Design review of the part built by this model. Coordinates are the model's own, in mm. Give positions to 0.01 mm unless a question says otherwise; leave off trailing zeros. Loops run counter-clockwise (first coordinate to the right, second up) from the corner with the lowest first, then second, coordinate; pieces in that order, holes last. Notation, with made-up numbers: (-5.75, 73.5) -> (42.25, 73.5) arc R22 cw to (42.25, 98.5) -> close; hole circle Ø5 at (-12, -4). An arc over 180 degrees is marked (long way). Use a Markdown table: item, result. Add a question column.
1. To check wall thickness, follow line 1 (X direction, y = 109, z = 10.1); line 2 (Z direction, x = 10.5, y = 164.5); line 3 (X direction, y = 16, z = 9). State the ranges of each line that lie inside material, in increasing order.
2. Add section D-D (y = 158). Count the separate pieces of the cut face and the enclosed holes in it, and give its area (3 significant figures).
3. Add section C-C (x = -10.1). State the section outline as (y, z) points.
4. Add section B-B (z = 10.1). State the section outline as (x, y) points, and give its area (3 significant figures).
5. Add section A-A (x = 0). State the section outline as (y, z) points, and give its area (3 significant figures).
6. For pin 1 Ø8 at (x, z) = (10.1, -10.1) entering from +Y; pin 2 Ø0.7 at (x, y) = (-14.5, 79.5) entering from +Z, all flat-tipped, find the tip position at first contact; note any pin that passes through.
```python
from build123d import *

# Parameters (mm, degrees)
SKETCH_1_R      = 2.5
SKETCH_1_R_2    = 3.4
EXTRUDE_1_DEPTH = 181


with BuildPart() as part:
    # 草图1 → 凸台-拉伸1 (new body)
    with BuildSketch(Plane(origin=(0, 0, 0), x_dir=(1, 0, 0), z_dir=(0, 1, 0))):
        with BuildLine():
            Line((-14, 15), (-3.25, 15))
            Line((-3.25, 15), (-3.25, 12.7))
            Line((-3.25, 12.7), (-5.2, 12.7))
            Line((-5.2, 12.7), (-5.2, 6.9))
            ThreePointArc((-5.2, 6.9), (0, 4.3), (5.2, 6.9))
            Line((5.2, 6.9), (5.2, 12.7))
            Line((5.2, 12.7), (3.25, 12.7))
            Line((3.25, 12.7), (3.25, 15))
            Line((3.25, 15), (14, 15))
            ThreePointArc((14, 15), (14.707106781, 14.707106781), (15, 14))
            Line((15, 14), (15, 3.25))
            Line((15, 3.25), (12.7, 3.25))
            Line((12.7, 3.25), (12.7, 5.2))
            Line((12.7, 5.2), (6.9, 5.2))
            ThreePointArc((6.9, 5.2), (4.3, 0), (6.9, -5.2))
            Line((6.9, -5.2), (12.7, -5.2))
            Line((12.7, -5.2), (12.7, -3.25))
            Line((12.7, -3.25), (15, -3.25))
            Line((15, -3.25), (15, -14))
            ThreePointArc((15, -14), (14.707106781, -14.707106781), (14, -15))
            Line((14, -15), (3.25, -15))
            Line((3.25, -15), (3.25, -12.7))
            Line((3.25, -12.7), (5.2, -12.7))
            Line((5.2, -12.7), (5.2, -6.9))
            ThreePointArc((5.2, -6.9), (0, -4.3), (-5.2, -6.9))
            Line((-5.2, -6.9), (-5.2, -12.7))
            Line((-5.2, -12.7), (-3.25, -12.7))
            Line((-3.25, -12.7), (-3.25, -15))
            Line((-3.25, -15), (-14, -15))
            ThreePointArc((-14, -15), (-14.707106781, -14.707106781), (-15, -14))
            Line((-15, -14), (-15, -3.25))
            Line((-15, -3.25), (-12.7, -3.25))
            Line((-12.7, -3.25), (-12.7, -5.2))
            Line((-12.7, -5.2), (-6.9, -5.2))
            ThreePointArc((-6.9, -5.2), (-4.3, 0), (-6.9, 5.2))
            Line((-6.9, 5.2), (-12.7, 5.2))
            Line((-12.7, 5.2), (-12.7, 3.25))
            Line((-12.7, 3.25), (-15, 3.25))
            Line((-15, 3.25), (-15, 14))
            ThreePointArc((-15, 14), (-14.707106781, 14.707106781), (-14, 15))
        make_face()
        with Locations(Location((0, 0, 0), (0, 0, 270))):
            Circle(SKETCH_1_R, mode=Mode.SUBTRACT)
        with Locations(Location((-10.1, 10.1, 0), (0, 0, 270))):
            Circle(SKETCH_1_R_2, mode=Mode.SUBTRACT)
        with Locations(Location((10.1, 10.1, 0), (0, 0, 90))):
            Circle(SKETCH_1_R_2, mode=Mode.SUBTRACT)
        with Locations(Location((10.1, -10.1, 0), (0, 0, 270))):
            Circle(SKETCH_1_R_2, mode=Mode.SUBTRACT)
        with Locations(Location((-10.1, -10.1, 0), (0, 0, 90))):
            Circle(SKETCH_1_R_2, mode=Mode.SUBTRACT)
    extrude(amount=EXTRUDE_1_DEPTH)


solid = part.part
```
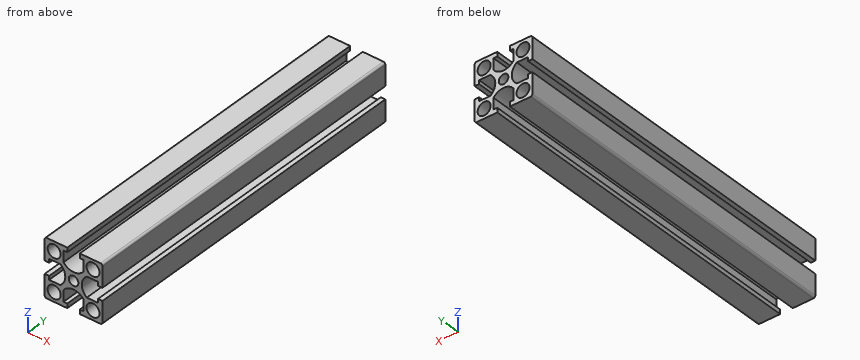
Taken from the geometry:
| question | item | result |
|---|---|---|
| 1 | line 1 | x = -15 to -13.5, -6.7 to -5.2, 5.2 to 6.7, 13.5 to 15 |
| 1 | line 2 | z = -15 to -13.48, -6.72 to -5.2, 5.2 to 6.72, 13.48 to 15 |
| 1 | line 3 | x = -15 to -13.32, -6.88 to -5.2, 5.2 to 6.88, 13.32 to 15 |
| 2 | separate pieces | 1 |
| 2 | enclosed holes | 5 |
| 2 | area | 358 mm^2 |
| 3 | outline | (0, -15) -> (181, -15) -> (181, -13.5) -> (0, -13.5) -> close; (0, -6.7) -> (181, -6.7) -> (181, -5.2) -> (0, -5.2) -> close; (0, 5.2) -> (181, 5.2) -> (181, 6.7) -> (0, 6.7) -> close; (0, 13.5) -> (181, 13.5) -> (181, 15) -> (0, 15) -> close |
| 4 | outline | (-15, 0) -> (-13.5, 0) -> (-13.5, 181) -> (-15, 181) -> close; (-6.7, 0) -> (-5.2, 0) -> (-5.2, 181) -> (-6.7, 181) -> close; (5.2, 0) -> (6.7, 0) -> (6.7, 181) -> (5.2, 181) -> close; (13.5, 0) -> (15, 0) -> (15, 181) -> (13.5, 181) -> close |
| 4 | area | 1,090 mm^2 |
| 5 | outline | (0, -4.3) -> (181, -4.3) -> (181, -2.5) -> (0, -2.5) -> close; (0, 2.5) -> (181, 2.5) -> (181, 4.3) -> (0, 4.3) -> close |
| 5 | area | 652 mm^2 |
| 6 | pin 1 | stops at y = 181 |
| 6 | pin 2 | stops at z = 14.99 |
